Geometry check sheet. Reference: the model listing, model coordinates, mm. A direction names the side the tool comes from. Coordinates: 2 decimals unless noted, no trailing zeros. Order: outer loops, then holes, each group sorted by start corner. A loop starts at its lowest first (then second) coordinate and runs counter-clockwise, first axis right, second up. Notation, with made-up numbers: (33.25, 81) - (60.25, 81) arc R26 cw to (60.25, 99) - close; hole circle Ø9 at (16.25, -34.5). An arc over 180 degrees is marked (long way). Put each result on its own line as item: value.
from build123d import *

# Parameters (mm, degrees)
BOSS_EXTRUDE3_DEPTH = 4
HOLE3_D             = 5.275
HOLE3_DEPTH         = 4
FILLET3_R           = 2
SKETCH25_R          = 1.506522666
BOSS_EXTRUDE4_DEPTH = 2


with BuildPart() as part:
    # Sketch17 → Boss-Extrude3 (new body)
    with BuildSketch(Plane(origin=(0, 0, 0), x_dir=(-1, 0, 0), z_dir=(0, 0, -1))):
        with BuildLine():
            Line((-43.273147001, 29.420937259), (-51.8645252, 33.076041142))
            ThreePointArc((-51.8645252, 33.076041142), (-60.191727201, 37.289326312), (-56.839071038, 28.579919803))
            Line((-56.839071038, 28.579919803), (-56.839071038, 23.292312115))
            Line((-56.839071038, 23.292312115), (-43.08257304, 23.292312115))
            ThreePointArc((-43.08257304, 23.292312115), (-34.429928081, 26.628647856), (-43.273147001, 29.420937259))
        make_face()
    extrude(amount=-BOSS_EXTRUDE3_DEPTH)

    # Hole3
    with Locations(Plane(origin=(0, 0, 0), x_dir=(-1, 0, 0), z_dir=(0, 0, -1))):
        with Locations((-39.340592987, 26.475947236), (-56.839071038, 33.579919803)):
            Hole(HOLE3_D / 2, depth=HOLE3_DEPTH)

    # Fillet3
    fillet3_edges = [part.edges().sort_by_distance(p)[0] for p in [
        (43.08257304, 23.292312115, 2),
        (56.839071038, 23.292312115, 2),
        (56.839071038, 28.579919803, 2),
        (51.8645252, 33.076041142, 2),
        (43.273147001, 29.420937259, 2),
    ]]
    fillet(fillet3_edges, radius=FILLET3_R)

    # Sketch25 → Boss-Extrude4 (add)
    with BuildSketch(Plane(origin=(47, 0, 0), x_dir=(0, 0, -1), z_dir=(1, 0, 0))):
        with BuildLine():
            Line((0, 23.292312115), (0, 30.144105031))
            add(Edge.make_bspline(
                [(2.034016737, 29.349553115), (0.844292257, 29.348828202), (0, 30.144105031)],
                knots=[0, 0, 0, 1, 1, 1], degree=2))
            ThreePointArc((2.034016737, 29.349553115), (4.534016737, 26.849553115), (2.034016737, 24.349553115))
            add(Edge.make_bspline(
                [(2.034016737, 24.349553115), (0.725821756, 24.359363318), (0, 23.292312115)],
                knots=[0, 0, 0, 1, 1, 1], degree=2))
        make_face()
        with Locations((2.034016737, 26.849553115)):
            Circle(SKETCH25_R, mode=Mode.SUBTRACT)
    extrude(amount=-BOSS_EXTRUDE4_DEPTH)


solid = part.part
Q1. Access from +Z, -Z, +X, -X, +Y, -Y to the whole of each face (thin tool, end or side, straight path). Record for faces 4 (the flat face through (56.839, 26, 2)), 5 (the flat face through (45, 25, -2)), 6 (the flat face through (47, 25, -2)).
Answer block:
face 4: +Z, -Z, +X, -Y
face 5: -Z, -X, +Y, -Y
face 6: -Z, +X, +Y, -Y
Q2. Section check D-D on x = 39.25. Record the boundary of the cut face in (y, z), then the cut area to 3 significant figures.
Answer block:
outline: (21.56, 0) - (23.84, 0) - (23.84, 4) - (21.56, 4) - close; (29.11, 0) - (31.39, 0) - (31.39, 4) - (29.11, 4) - close
area: 18.2 mm^2
Q3. Depth check by flat-ended pin: pin 1 Ø10 at (x, y) = (57, 36.5) entering from -Z; pin 2 Ø1.2 at (x, z) = (48, 2.5) entering from -Y; pin 3 Ø3.5 at (y, z) = (27, -2) entering from +X. Enter the tip coordinate at first touch or a pass-through.
Answer block:
pin 1: stops at z = 0
pin 2: stops at y = 23.29
pin 3: stops at x = 47
Q4. Section check B-B on z = -2.5. Record the boundary of the cut face in (x, y).
Answer block:
outline: (45, 24.39) - (47, 24.39) - (47, 25.42) - (45, 25.42) - close; (45, 28.28) - (47, 28.28) - (47, 29.31) - (45, 29.31) - close
Q5. Section check C-C on y = 25. Record the boundary of the cut face in (x, z).
Answer block:
outline: (34.65, 0) - (37.15, 0) - (37.15, 4) - (34.65, 4) - close; (41.53, 0) - (45, 0) - (45, -3.72) - (47, -3.72) - (47, 0) - (56.82, 0) - (56.82, 4) - (41.53, 4) - close
Q6. Section check A-A on y = 27.5. Record the boundary of the cut face in (x, z).
Answer block:
outline: (34.54, 0) - (36.91, 0) - (36.91, 4) - (34.54, 4) - close; (41.77, 0) - (45, 0) - (45, -0.68) - (47, -0.68) - (47, 0) - (56.94, 0) - (56.94, 4) - (41.77, 4) - close; (45, -4.45) - (47, -4.45) - (47, -3.39) - (45, -3.39) - close
Q7. Draft check along Z on faces 1 (the cylindrical face through (46.014, 26.905, -4.533)), 2 (the flat face through (47.56, 31.245, 1.972)), 3 (the cylindrical face through (46.014, 28.343, -1.838)). Enter one of: pulls with the +Z half, pulls with the -Z half, needs draft (parallel to the pull), parting line crosses it, or undercut.
Answer block:
face 1: pulls with the -Z half
face 2: needs draft
face 3: undercut
Q8. Thickness scan on L1, parallel to Z at x = 42.25, y = 30; L2, parallel to X at y = 25.25, z = 2; L3, parallel to X at y = 27, z = 0.75. Record the ranges inside material, lowest first. Write a range as [from, to].
Answer block:
L1: z = [0, 4]
L2: x = [34.58, 37.01], [41.68, 56.84]
L3: x = [34.46, 36.76], [41.93, 56.84]
